from build123d import *

# Parameters (mm, degrees)
F1_DEPTH  = 2
F3_DEPTH  = 4
F4_W      = 0.5
F4_H      = 15
F5_DEPTH  = 25
F6_DEPTH  = 2
F8_DEPTH  = 25
F10_DEPTH = 25


with BuildPart() as f1:
    # F0 (on Top) → F1 (new body)
    with BuildSketch(Plane.XY):
        Polygon((-7.4135116758, 0), (-0.25, -15.362200364), (-0.25, -5.8973940314), (-3, 0), (-14.3537370712, 24.3481677229), (-17.9789682194, 22.6576946759), align=None)
        Polygon((0.25, -15.362200364), (7.4135116758, 0), (17.9789682194, 22.6576946759), (14.3537370712, 24.3481677229), (3, 0), (0.25, -5.8973940314), align=None)
        Polygon((0, -15.8983270941), (0.25, -15.362200364), (0.25, -5.8973940314), (0, -6.4335207615), (-0.25, -5.8973940314), (-0.25, -15.362200364), align=None)
    extrude(amount=F1_DEPTH)

    # F2 (on face) → F3 (join)
    with BuildSketch(Plane.XY.offset(2)):
        with BuildLine():
            ThreePointArc((-8.8668911775, 12.581588732), (0, 9.4157126397), (8.8668911775, 12.581588732))
            Line((8.8668911775, 12.581588732), (9.6599709615, 14.2823538173))
            ThreePointArc((9.6599709615, 14.2823538173), (0, 10.4157126397), (-9.6599709615, 14.2823538173))
            Line((-9.6599709615, 14.2823538173), (-8.8668911775, 12.581588732))
        make_face()
        with BuildLine():
            ThreePointArc((-13.9989482009, 23.5873205351), (-12.6883090185, 17.4990569753), (-8.8668911775, 12.581588732))
            Line((-8.8668911775, 12.581588732), (-9.6599709615, 14.2823538173))
            ThreePointArc((-9.6599709615, 14.2823538173), (-12.6883090185, 18.4990569753), (-13.97191286, 23.5293430595))
            Line((-13.97191286, 23.5293430595), (-13.9989482009, 23.5873205351))
        make_face()
        with BuildLine():
            ThreePointArc((-13.97191286, 23.5293430595), (-12.6883090185, 18.4990569753), (-9.6599709615, 14.2823538173))
            Line((-9.6599709615, 14.2823538173), (-13.97191286, 23.5293430595))
        make_face()
    extrude(amount=-F3_DEPTH)

    # F4 (on face) → F5 (cut)
    with BuildSketch(Plane.XY.offset(2)):
        with Locations((0, -9.3687182158)):
            Rectangle(F4_W, F4_H)
    extrude(amount=-F5_DEPTH, mode=Mode.SUBTRACT)

    # F6 (add): faces of the model
    f6_faces = [f1.faces().sort_by_distance(p)[0] for p in [
        (-7.9421134858, 5.393960994, 0),
        (8.2425809304, 6.3306998172, 0),
    ]]
    extrude(f6_faces, amount=F6_DEPTH)

    # F7 (on face) → F8 (join)
    with BuildSketch(Plane.XY.offset(2)):
        Polygon((-0.25, -5.8973940314), (-2.7857095704, -0.4595473092), (-2.7857095704, -9.9243536418), (-0.25, -15.362200364), align=None)
        Polygon((2.7857095704, -9.9243536418), (2.7857095704, -0.4595473092), (0.25, -5.8973940314), (0.25, -15.362200364), align=None)
    extrude(amount=F8_DEPTH)

    # F9 (on face) → F10 (join)
    with BuildSketch(Plane(origin=(0, 0, -2), x_dir=(1, 0, 0), z_dir=(0, 0, -1))):
        Polygon((-0.25, 15.362200364), (-2.7857095704, 9.9243536418), (-2.7857095704, 0.4595473092), (-0.25, 5.8973940314), align=None)
        Polygon((0.25, 5.8973940314), (2.7857095704, 0.4595473092), (2.7857095704, 9.9243536418), (0.25, 15.362200364), align=None)
    extrude(amount=F10_DEPTH)


solid = f1.part
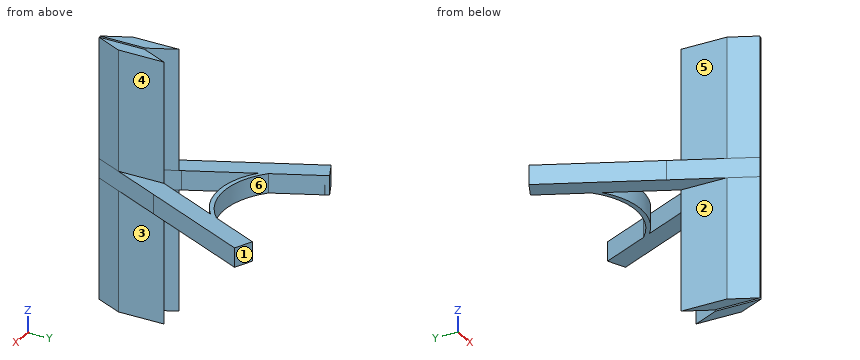
Source: CAD feature listing. Evaluate the final solid. Frame: model axes, mm. Face numbers are marked on the shaded views. A direction names the side the tool comes from. Round coordinates to 2 decimals unless told otherwise and drop trailing zeros. Loops run counter-clockwise (first coordinate to the right, second up) from the corner with the lowest first, then second, coordinate; pieces in that order, holes last.
Q1. Section B-B, the plane y = -4. Return loops of the section in (x, z), plus the area to 3 significant figures.
Q2. Access query for the marked faces 1, 2 and 3. Directions: +Z, -Z, +X, -X, +Y, -Y. A direction counts if a zero-diameter tool reaches every point of the face in a straight line with its end or side. Return the directions, or none.
Q3. Section A-A, the plane z = -21. Return loops of the section in (x, y).
Q4. Section D-D, the plane y = -8. Return loops of the section in (x, z).
Q5. Section C-C, the plane x = -5. Return loops of the section in (y, z), plus the area to 3 significant figures.
Q6. Ray query, line 1 (X direction, y = -9, z = -23.5); line 2 (Y direction, x = 3, z = -1); line 3 (X direction, y = -1, z = 8.5). Return the intervals inside material, ascending.
Q7. First-contact query: P1, Ø1.5, axis at x = -12.5, y = 15, coming from the +Z side; P2, Ø10.5, axis at y = -6, z = -13, coming from the -X side; P3, Ø5, axis at y = 14, z = -2, coming from the +X side; P4, Ø10, axis at x = -7, y = -7.5, coming from the -Z side. Flat tips, straight axial feed; report the tip coordinate or a pass-through.
Q8. Mould query, pull axis X, two halves, no side actions, for the marked faces 4, 5 and 6. Classes: pulls with the +X half, pulls with the -X half, needs draft (parallel to the pull), parting line crosses it, or undercut.
Solutions:
1. outline: (-5.55, -2) - (-2.79, -2) - (-2.79, -27) - (-1.13, -27) - (-1.13, 27) - (-2.79, 27) - (-2.79, 2) - (-5.55, 2) - close; (1.13, -27) - (2.79, -27) - (2.79, -2) - (5.55, -2) - (5.55, 2) - (2.79, 2) - (2.79, 27) - (1.13, 27) - close
1. area: 200 mm2
2. face 1: +Z, -Z, +X, +Y
2. face 2: -Z, -X, +Y, -Y
2. face 3: -Z, +X, +Y, -Y
3. outline: (-2.79, -9.92) - (-0.25, -15.36) - (-0.25, -5.9) - (-2.79, -0.46) - close; (0.25, -15.36) - (2.79, -9.92) - (2.79, -0.46) - (0.25, -5.9) - close
4. outline: (-3.68, -2) - (-2.79, -2) - (-2.79, -27) - (-0.25, -27) - (-0.25, 27) - (-2.79, 27) - (-2.79, 2) - (-3.68, 2) - close; (0.25, -27) - (2.79, -27) - (2.79, -2) - (3.68, -2) - (3.68, 2) - (2.79, 2) - (2.79, 27) - (0.25, 27) - close
5. outline: (-5.18, -2) - (4.29, -2) - (4.29, 2) - (-5.18, 2) - close; (10.34, -2) - (11.34, -2) - (11.34, 2) - (10.34, 2) - close
5. area: 41.9 mm2
6. line 1: x = -2.79 to -0.25, 0.25 to 2.79
6. line 2: y = -9.46 to 0, 9.74 to 10.74
6. line 3: x = -2.79 to -2.53, 2.53 to 2.79
7. P1: stops at z = 2
7. P2: stops at x = -2.79
7. P3: stops at x = 15.11
7. P4: stops at z = -27
8. face 4: pulls with the +X half
8. face 5: pulls with the -X half
8. face 6: undercut
